```python
from build123d import *

# Parameters (mm, degrees)
F0_R     = 2
F1_DEPTH = 3.5
F4_SIZE  = 0.3


with BuildPart() as f1:
    # F0 (on Top) → F1 (new body)
    with BuildSketch(Plane.XY):
        Polygon((3.031089, 1.75), (0, 3.5), (-3.031089, 1.75), (-3.031089, -1.75), (0, -3.5), (3.031089, -1.75), align=None)
        Circle(F0_R, mode=Mode.SUBTRACT)
    extrude(amount=F1_DEPTH)

    # F2 (on Front) → F3 (revolve, cut)
    with BuildSketch(Plane.XZ):
        Polygon((3.031089, 3.5), (5.80237, 1.9), (5.80237, 3.5), align=None)
        Polygon((5.80237, 1.6), (3.031089, 0), (5.80237, 0), align=None)
    revolve(axis=Axis((0, 0, 1.75), (0, 0, -1)), mode=Mode.SUBTRACT)

    # F4
    f4_edges = [f1.edges().sort_by_distance(p)[0] for p in [
        (-2, 0, 3.5),
        (-2, 0, 0),
    ]]
    chamfer(f4_edges, length=F4_SIZE)


solid = f1.part
```
CAD build for the part. Positions are in the model's coordinates, mm. Coordinates: 2 decimals unless noted, no trailing zeros. Loops run counter-clockwise (first coordinate to the right, second up) from the corner with the lowest first, then second, coordinate; pieces in that order, holes last. Notation, with made-up numbers: (33, 50) - (44, 50) arc R37 cw to (44, 88) - close; hole circle Ø7 at (67.5, -1.5). An arc over 180 degrees is marked (long way). Return JSON: item names as keys, results as strings.
1. Mould opens along X. For faces 1 (the flat face through (-2, 2, 0)), 2 (the flat face through (-1.54, -2.61, 1.73)), 3 (the cylindrical face through (0, -2, 2)) say: released by +X, released by -X, zero draft, split by the parting line, or undercut.
Result:
{"face 1": "zero draft", "face 2": "released by -X", "face 3": "undercut"}
2. Band-saw the part on A-A (z = 1.1). Give the cut face in (x, y), and give its area (3 significant figures).
Result:
{"outline": "(-3.03, -1.75) - (0, -3.5) - (3.03, -1.75) - (3.03, 1.75) - (0, 3.5) - (-3.03, 1.75) - close; hole circle Ø4 at (0, 0)", "area": "19.3 mm2"}
3. Drop flat-ended pins along their axis: pin 1 (2 mm diameter, centred on x = 2, z = 0.5, fed in from +Y); pin 2 (1 mm diameter, centred on x = 1, z = 1.5, fed in from -Y); pin 3 (2 mm diameter, centred on x = 0.5, z = 1.5, fed in from -Y); pin 4 (3 mm diameter, centred on x = -2.5, y = -2.5, fed in from -Z). Give the stop position or say it passes through.
Result:
{"pin 1": "stops at y = 2.92", "pin 2": "stops at y = -3.21", "pin 3": "stops at y = -3.5", "pin 4": "stops at z = 0"}
4. Probe L1, parallel to X at y = -1.5, z = 2.9; L2, parallel to Y at x = 0.25, z = 0.8; L3, parallel to X at y = 0.75, z = 1.7. List the from-to ranges inside material, lowest first. Write a range as from..to.
Result:
{"L1": "x = -3.03..-1.32, 1.32..3.03", "L2": "y = -3.36..-1.98, 1.98..3.36", "L3": "x = -3.03..-1.85, 1.85..3.03"}
